Read the model definition and answer for the solid it produces. Units are mm, in the model's axes. A direction names the side the tool comes from. Give positions to 0.01 mm unless a question says otherwise; leave off trailing zeros. Loops run counter-clockwise (first coordinate to the right, second up) from the corner with the lowest first, then second, coordinate; pieces in that order, holes last. Notation, with made-up numbers: (-23.75, 54) - (23.25, 54) arc R23 cw to (23.25, 87) - close; hole circle Ø4 at (40, 5.25). An arc over 180 degrees is marked (long way). Put each result on its own line as item: value. Start each with the question number.
1. For faces 4 (the cylindrical face through (-100.504, 0.198, 3.479)), 5 (the flat face through (-49, 0, 5)), 6 (the cylindrical face through (5, 19, 1)), determine the directions among +Z, -Z, +X, -X, +Y, -Y from which every point of the face is accessible in a straight line to the end or side of a thin tool.
2. A cutting plane is placed at A-A, the plane y = -8.5. Determine the outline of the cut face in (x, z), plus the area to 3 significant figures.
3. A cutting plane is placed at D-D, the plane z = 10. Determine the outline of the cut face in (x, y).
4. For a pull along Y with two mould halves and no side action, classify faces 1 (the cylindrical face through (5.59, 4.46, 3.48)), 2 (the flat face through (-14, 0, 23)), 3 (the cylindrical face through (-49.3, 0.55, 24.994)) as released by +Y, released by -Y, zero draft, split by the parting line, or undercut.
5. Consider L1, parallel to Z at x = -95.5, y = -0.5 (3 decimals); L2, parallel to Y at x = -105, z = 3; L3, parallel to Y at x = 5, z = 4.65. Determine where each line is inside the solid, lowest interval first. Write a range as from..to.
6. Given pin 1 Ø4 at (x, z) = (-78, 12) entering from -Y; pin 2 Ø0.6 at (x, y) = (5.5, -16.5) entering from -Z; pin 3 Ø3 at (y, z) = (19.5, 15) entering from +X, each flat-ended and moving along its own axis, determine where each tip first touches the part or whether it passes through.
7. A cutting plane is placed at C-C, the plane z = 3.5. Count the separate pieces of the cut face and the enclosed holes in it, plus the area to 3 significant figures.
8. A cutting plane is placed at B-B, the plane x = -23. Determine the outline of the cut face in (y, z), plus the area to 3 significant figures.
```python
from build123d import *

# Parameters (mm, degrees)
REVOLVE1_ANGLE          = 180
SKETCH7_R               = 4.5
CUT_EXTRUDE2_DEPTH      = 26
CUT_EXTRUDE5_DEPTH      = 26
CUT_EXTRUDE5_DEPTH_BACK = 126
SKETCH12_W              = 5
SKETCH12_H              = 50
CUT_EXTRUDE6_DEPTH      = 20
CUT_EXTRUDE6_DEPTH_BACK = 30
CUT_EXTRUDE7_START      = -5
CUT_EXTRUDE7_DEPTH      = 2
SKETCH14_R              = 1
CUT_EXTRUDE8_DEPTH      = 5


with BuildPart() as part:
    # Sketch5 → Revolve1 (revolve)
    with BuildSketch(Plane.XY):
        with BuildLine():
            Line((0, 0), (-100, 0))
            Line((-100, 0), (-125, 0))
            ThreePointArc((-125, 0), (-117.67766953, 17.67766953), (-100, 25))
            Line((-100, 25), (0, 25))
            ThreePointArc((0, 25), (17.67766953, 17.67766953), (25, 0))
            Line((25, 0), (0, 0))
        make_face()
    revolve(axis=Axis((-64.676616915, 0, 0), (1, 0, 0)), revolution_arc=REVOLVE1_ANGLE)

    # Sketch7 → Cut-Extrude2 (cut, through all)
    with BuildSketch(Plane(origin=(0, 0, 0), x_dir=(-1, 0, 0), z_dir=(0, 0, -1))):
        with Locations((-5, 0)):
            Circle(SKETCH7_R)
        with Locations((105, 0)):
            Circle(SKETCH7_R)
    extrude(amount=-CUT_EXTRUDE2_DEPTH, mode=Mode.SUBTRACT)

    # Sketch10 → Cut-Extrude5 (cut, two sides)
    with BuildSketch(Plane(origin=(0, 0, 0), x_dir=(0, 0, -1), z_dir=(1, 0, 0))) as cut_extrude5_sk:
        with BuildLine():
            Line((-5, 15), (-5, -15))
            ThreePointArc((-5, -15), (-20, 0), (-5, 15))
        make_face()
    extrude(amount=CUT_EXTRUDE5_DEPTH, mode=Mode.SUBTRACT)
    extrude(cut_extrude5_sk.sketch, amount=-CUT_EXTRUDE5_DEPTH_BACK, mode=Mode.SUBTRACT)

    # Sketch12 → Cut-Extrude6 (cut, two sides)
    with BuildSketch(Plane(origin=(0, 0, 0), x_dir=(0, 0, -1), z_dir=(1, 0, 0))) as cut_extrude6_sk:
        with Locations((-25.5, 0)):
            Rectangle(SKETCH12_W, SKETCH12_H)
    extrude(amount=CUT_EXTRUDE6_DEPTH, mode=Mode.SUBTRACT)
    extrude(cut_extrude6_sk.sketch, amount=-CUT_EXTRUDE6_DEPTH_BACK, mode=Mode.SUBTRACT)

    # Sketch13 → Cut-Extrude7 (cut)
    with BuildSketch(Plane.XY.offset(5).offset(CUT_EXTRUDE7_START)):
        with BuildLine():
            Line((7.5, 16.5), (8.79175539, 6.456036683))
            ThreePointArc((8.79175539, 6.456036683), (9.53927005, 4.651376653), (11.34393008, 3.903861993))
            add(Edge.make_bspline(
                [(21.5, 2.5), (11.34393008, 3.903861993)],
                knots=[0, 0, 1, 1], degree=1))
            ThreePointArc((21.5, 2.5), (24, 0), (21.5, -2.5))
            Line((21.5, -2.5), (11.456036683, -3.79175539))
            ThreePointArc((11.456036683, -3.79175539), (9.651376653, -4.53927005), (8.903861993, -6.34393008))
            Line((8.903861993, -6.34393008), (7.5, -16.5))
            ThreePointArc((7.5, -16.5), (5, -19), (2.5, -16.5))
            Line((2.5, -16.5), (1.20824461, -6.456036683))
            ThreePointArc((1.20824461, -6.456036683), (0.46072995, -4.651376653), (-1.34393008, -3.903861993))
            Line((-1.34393008, -3.903861993), (-11.5, -2.5))
            ThreePointArc((-11.5, -2.5), (-14, 0), (-11.5, 2.5))
            Line((-11.5, 2.5), (-1.456036683, 3.79175539))
            ThreePointArc((-1.456036683, 3.79175539), (0.348623347, 4.53927005), (1.096138007, 6.34393008))
            Line((1.096138007, 6.34393008), (2.5, 16.5))
            ThreePointArc((2.5, 16.5), (5, 19), (7.5, 16.5))
        make_face()
        with BuildLine():
            Line((-102.5, 16.5), (-101.127521023, 6.403861993))
            ThreePointArc((-101.127521023, 6.403861993), (-100.395287976, 4.63609504), (-98.627521023, 3.903861993))
            add(Edge.make_bspline(
                [(-88.5, 2.5), (-98.627521023, 3.903861993)],
                knots=[0, 0, 1, 1], degree=1))
            ThreePointArc((-88.5, 2.5), (-86, 0), (-88.5, -2.5))
            Line((-88.5, -2.5), (-98.627521023, -3.79175539))
            ThreePointArc((-98.627521023, -3.79175539), (-100.395287976, -4.523988437), (-101.127521023, -6.29175539))
            Line((-101.127521023, -6.29175539), (-102.5, -16.5))
            ThreePointArc((-102.5, -16.5), (-105, -19), (-107.5, -16.5))
            Line((-107.5, -16.5), (-108.823138405, -6.29175539))
            ThreePointArc((-108.823138405, -6.29175539), (-109.555371452, -4.523988437), (-111.323138405, -3.79175539))
            Line((-111.323138405, -3.79175539), (-121.5, -2.5))
            ThreePointArc((-121.5, -2.5), (-124, 0), (-121.5, 2.5))
            Line((-121.5, 2.5), (-111.323138405, 3.903861993))
            ThreePointArc((-111.323138405, 3.903861993), (-109.555371452, 4.63609504), (-108.823138405, 6.403861993))
            Line((-108.823138405, 6.403861993), (-107.5, 16.5))
            ThreePointArc((-107.5, 16.5), (-105, 19), (-102.5, 16.5))
        make_face()
    extrude(amount=CUT_EXTRUDE7_DEPTH, mode=Mode.SUBTRACT)

    # Sketch14 → Cut-Extrude8 (cut)
    with BuildSketch(Plane(origin=(0, 0, 2), x_dir=(-1, 0, 0), z_dir=(0, 0, -1))):
        with Locations((-5, 16.5)):
            Circle(SKETCH14_R)
        with Locations((11.5, 0)):
            Circle(SKETCH14_R)
        with Locations((-5, -16.5)):
            Circle(SKETCH14_R)
        with Locations((-21.5, 0)):
            Circle(SKETCH14_R)
        with Locations((105, 16.5)):
            Circle(SKETCH14_R)
        with Locations((121.5, 0)):
            Circle(SKETCH14_R)
        with Locations((105, -16.5)):
            Circle(SKETCH14_R)
        with Locations((88.5, 0)):
            Circle(SKETCH14_R)
    extrude(amount=-CUT_EXTRUDE8_DEPTH, mode=Mode.SUBTRACT)


solid = part.part
```
Return value:
1. face 4: +Z, -Z
1. face 5: +X, -X
1. face 6: -Z
2. outline: (-123.51, 0) - (-108.54, 0) - (-108.54, 2) - (-101.42, 2) - (-101.42, 0) - (1.47, 0) - (1.47, 2) - (8.61, 2) - (8.61, 0) - (23.51, 0) arc R23.51 ccw to (22.97, 5) - (-122.97, 5) arc R23.51 ccw to start; (-115.86, 17.36) - (15.86, 17.36) arc R23.51 ccw to (4.87, 23) - (-30, 23) - (-30, 23.51) - (-100, 23.51) arc R23.51 ccw to start
2. area: 1,440 mm2
3. outline: (-118.03, -14.14) arc R22.91 ccw to (-100, -22.91) - (0, -22.91) arc R22.91 ccw to (18.03, -14.14) - close; (-118.03, 14.14) - (18.03, 14.14) arc R22.91 ccw to (0, 22.91) - (-100, 22.91) arc R22.91 ccw to start
4. face 1: undercut
4. face 2: zero draft
4. face 3: split by the parting line
5. L1: z = 2..5, 19.992..24.995
5. L2: y = -24.31..-17.5, -15.5..-4.5, 4.5..15.5, 17.5..24.31
5. L3: y = -24.05..-17.5, -15.5..-4.5, 4.5..15.5, 17.5..24.05
6. pin 1: stops at y = -22.91
6. pin 2: stops at z = 7
6. pin 3: stops at x = 9.56
7. separate pieces: 1
7. enclosed holes: 10
7. area: 6,720 mm2
8. outline: (-25, 0) - (25, 0) arc R25 ccw to (9.8, 23) - (-9.8, 23) arc R25 ccw to start; hole (-15, 5) - (15, 5) arc R15 ccw to start
8. area: 602 mm2
